Could you check a few things on this model? Use its own coordinates, in mm. A direction names the side the tool comes from. Coordinates: 2 decimals unless noted, no trailing zeros. Write each loop counter-clockwise with the first axis right and the second up, starting at its lowest first coordinate (ties: lowest second). Pieces come first, ordered by that corner, then holes.
Item 1: Which directions (+Z, -Z, +X, -X, +Y, -Y) give clear straight access to the entire face, cutting with the end or side of a thin tool? Please do faces 1 (the flat face through (6, -17, 87.403)), 2 (the flat face through (6, -42.119, 5)).
Item 2: I want a section at B-B on z = 69. Please give me the cut outline in (x, y).
Item 3: For P1, Ø4, axis at x = 1.5, z = -16, coming from the +Y side; P2, Ø4, axis at x = 2.5, z = -36, coming from the +Y side, each with a flat end and sliding along its axis, tell me the tip position at first contact or that it passes through.
Item 4: If I drill on probe 1 along Z at (x, y) = (9.5, 4.5); probe 2 along Y at (x, z) = (8, -35); probe 3 along Y at (x, z) = (3, -5.5), over which ranges is the centre line in solid material (lowest first)?
Item 5: Thinking about a two-plate mould opening in Z: for faces 3 (the flat face through (12, -41, 4)), 4 (the flat face through (6, -17, 89.403)), 5 (the flat face through (7, 5.281, 2)), which applies, +Z half, -Z half, draft (parallel to the pull), parting line (faces both ways), or undercut?
Item 6: I want a section at A-A on y = -14.5. Please give me the cut outline in (x, z), then the cut area to 3 significant figures.
Autodesk Inventor part; units mm, degrees
ref_plane "YZ Plane" through (0, 0, 0) normal (1, 0, 0) x (0, 1, 0)
ref_plane "XZ Plane" through (0, 0, 0) normal (0, 1, 0) x (-1, 0, 0)
ref_plane "XY Plane" through (0, 0, 0) normal (0, 0, 1) x (1, 0, 0)
sketch "Sketch1" plane through (0, 0, 0) normal (1, 0, 0) x (0, 1, 0)
  line L0 (5.2806, 87.403) -> (-40.1194, 87.403)
  line L1 (-40.1194, 87.403) -> (-40.1194, -80.597)
  line L2 (-40.1194, -80.597) -> (5.2806, -80.597)
  line L3 (5.2806, -80.597) -> (5.2806, 87.403)
  line L4 (7.2806, 89.403) -> (-42.1194, 89.403)
  line L5 (-42.1194, 89.403) -> (-42.1194, -82.597)
  line L6 (-42.1194, -82.597) -> (7.2806, -82.597)
  line L7 (7.2806, -82.597) -> (7.2806, 89.403)
  point P0 (0, 0)
  dimension "d0" = 168
  dimension "d1" = 45.4
  dimension "d2" = 2
extrude "Extrusion1" add sketch "Sketch1" along normal blind 12
sketch "Sketch2" plane through (0, 7.2806, 89.403) normal (0, 1, 0) x (1, 0, 0)
  line L0 (12, 172) -> (12, 0)
  line L1 (0, 0) -> (12, 0)
  point P0 (0, 89.403)
  point P1 (6, 8)
  dimension "d5" = 6
  dimension "d6" = 8
hole "Hole1" at (6, 7.2806, 81.403) direction (0, -1, 0) diameter 4 depth 10 tip angle 118 countersink diameter 8.4 countersink angle 90
ref_plane "Work Plane1" through (0, -42.1194, 3.403) normal (0, 0, 1) x (1, 0, 0)
mirror "Mirror1" about plane through (0, -42.1194, 3.403) normal (0, 0, 1) of "Hole1"
sketch "Sketch3" plane through (0, 7.2806, 89.403) normal (0, 1, 0) x (1, 0, 0)
  line L0 (0, 0) -> (0, 172)
  line L1 (0, 16) -> (4, 16)
  line L2 (4, 16) -> (4, 156)
  line L3 (4, 156) -> (0, 156)
  line L4 (0, 156) -> (0, 16)
  line L5 (0, 0) -> (12, 0)
  line L6 (0, 172) -> (12, 172)
  circle A0 centre (6, 8) radius 2.2
  point P0 (0, 89.403)
  point P1 (0, 156)
  dimension "d15" = 16
  dimension "d16" = 4
  dimension "d22" = 8
  dimension "d23" = 8
extrude "Extrusion2" cut sketch "Sketch3" against normal blind 10 contours L0 L3 L2 L1
chamfer "Chamfer1" distance 1.5 angle 45 5 edges at (4, 7.2806, 3.403) (2, 7.2806, 73.403) (0, 7.2806, 81.403) (2, 7.2806, -66.597) (0, 7.2806, -74.597)
sketch "Sketch4" plane through (12, 0, 0) normal (1, 0, 0) x (0, 0, -1)
  point P0 (0, 0)
sketch "Sketch5" plane through (0, -42.1194, -82.597) normal (0, -1, 0) x (1, 0, 0)
  circle A0 centre (6, 164) radius 2.2
  circle A1 centre (6, 8) radius 2.2
  point P0 (0, 82.597)
hole "Hole2" at (6, -42.1194, 81.403) at (6, -42.1194, -74.597) direction (0, 1, 0) diameter 4 depth 10 tip angle 118 countersink diameter 8.4 countersink angle 90
properties part number "front ring part"
Response values:
1. face 1: +X, -X
1. face 2: +Z, -Z, +X, -X, -Y
2. outline: (0, -42.12) - (12, -42.12) - (12, -40.12) - (0, -40.12) - close; (4, 5.28) - (12, 5.28) - (12, 7.28) - (5.5, 7.28) - (4, 5.78) - close
3. P1: stops at y = -40.12
3. P2: stops at y = 6.28
4. probe 1: z = -82.6 to -80.6, 87.4 to 89.4
4. probe 2: y = -42.12 to -40.12, 5.28 to 7.28
4. probe 3: y = -42.12 to -40.12
5. face 3: draft
5. face 4: +Z half
5. face 5: undercut
6. outline: (0, -82.6) - (12, -82.6) - (12, -80.6) - (0, -80.6) - close; (0, 87.4) - (12, 87.4) - (12, 89.4) - (0, 89.4) - close
6. area: 48.0 mm2
